Model file for the job. Use its own axes, mm. A direction names the side the tool comes from. Round coordinates to 2 decimals unless told otherwise and drop trailing zeros. Write each loop counter-clockwise with the first axis right and the second up, starting at its lowest first coordinate (ties: lowest second). Pieces come first, ordered by that corner, then holes. Notation, with made-up numbers: (16.25, 21.25) - (52.25, 21.25) arc R27 ccw to (52.25, 46.25) - close; hole circle Ø10 at (25.5, -39). An arc over 180 degrees is marked (long way). One line per item, written item: value.
from build123d import *

# Parameters (mm, degrees)
SKETCH1_W                                        = 192.5
SKETCH1_H                                        = 55
BOSS_EXTRUDE1_DEPTH                              = 20
CBORE_FOR_M4_HEX_HEAD_MACHINE_SCREW1_D           = 4.5
CBORE_FOR_M4_HEX_HEAD_MACHINE_SCREW1_DEPTH       = 55
CBORE_FOR_M4_HEX_HEAD_MACHINE_SCREW1_CBORE_D     = 9
CBORE_FOR_M4_HEX_HEAD_MACHINE_SCREW1_CBORE_DEPTH = 50
CBORE_FOR_M4_HEX_HEAD_MACHINE_SCREW2_D           = 4.5
CBORE_FOR_M4_HEX_HEAD_MACHINE_SCREW2_DEPTH       = 20
CBORE_FOR_M4_HEX_HEAD_MACHINE_SCREW2_CBORE_D     = 9
CBORE_FOR_M4_HEX_HEAD_MACHINE_SCREW2_CBORE_DEPTH = 5
CHAMFER1_SIZE                                    = 1


with BuildPart() as part:
    # Sketch1 → Boss-Extrude1 (new body)
    with BuildSketch(Plane(origin=(0, 0, 0), x_dir=(-1, 0, 0), z_dir=(0, 0, -1))):
        with Locations((-96.25, 27.5)):
            Rectangle(SKETCH1_W, SKETCH1_H)
    extrude(amount=-BOSS_EXTRUDE1_DEPTH)

    # CBORE for M4 Hex Head Machine Screw1
    with Locations(Plane(origin=(0, 0, 0), x_dir=(-1, 0, 0), z_dir=(0, -1, 0))):
        with Locations((-110, -10), (-10, -10)):
            CounterBoreHole(CBORE_FOR_M4_HEX_HEAD_MACHINE_SCREW1_D / 2, CBORE_FOR_M4_HEX_HEAD_MACHINE_SCREW1_CBORE_D / 2, CBORE_FOR_M4_HEX_HEAD_MACHINE_SCREW1_CBORE_DEPTH, depth=CBORE_FOR_M4_HEX_HEAD_MACHINE_SCREW1_DEPTH)

    # CBORE for M4 Hex Head Machine Screw2
    with Locations(Plane(origin=(0, 0, 0), x_dir=(-1, 0, 0), z_dir=(0, 0, -1))):
        with Locations((-182.5, 38), (-32.5, 38)):
            CounterBoreHole(CBORE_FOR_M4_HEX_HEAD_MACHINE_SCREW2_D / 2, CBORE_FOR_M4_HEX_HEAD_MACHINE_SCREW2_CBORE_D / 2, CBORE_FOR_M4_HEX_HEAD_MACHINE_SCREW2_CBORE_DEPTH, depth=CBORE_FOR_M4_HEX_HEAD_MACHINE_SCREW2_DEPTH)

    # Chamfer1
    chamfer1_edges = [part.edges().sort_by_distance(p)[0] for p in [
        (192.5, 27.5, 20),
        (96.25, 0, 20),
        (0, 27.5, 20),
        (96.25, 0, 0),
        (192.5, 27.5, 0),
        (96.25, 55, 0),
        (0, 27.5, 0),
        (0, 0, 10),
        (192.5, 0, 10),
        (192.5, 55, 10),
        (0, 55, 10),
        (96.25, 55, 20),
    ]]
    chamfer(chamfer1_edges, length=CHAMFER1_SIZE)


solid = part.part
1. Band-saw the part on B-B on y = 38. Write the cut outline in (x, z).
Report:
outline: (0, 1) - (1, 0) - (28, 0) - (28, 5) - (30.25, 5) - (30.25, 20) - (1, 20) - (0, 19) - close; (34.75, 5) - (37, 5) - (37, 0) - (178, 0) - (178, 5) - (180.25, 5) - (180.25, 20) - (34.75, 20) - close; (184.75, 5) - (187, 5) - (187, 0) - (191.5, 0) - (192.5, 1) - (192.5, 19) - (191.5, 20) - (184.75, 20) - close; hole circle Ø9 at (10, 10); hole circle Ø9 at (110, 10)
2. Mould opens along X. For faces 4 (the face through (98, 55, 10)), 5 (the face through (114.496, 24.65, 9.802)), 6 (the face through (192.5, 27, 10)), 7 (the face through (0, 27, 10)) say: released by +X, released by -X, zero draft, split by the parting line, or undercut.
Report:
face 4: zero draft
face 5: undercut
face 6: released by +X
face 7: released by -X
3. Band-saw the part on A-A on x = 32.5. Write the cut outline in (y, z), plus the area to 4 significant figures.
Report:
outline: (0, 1) - (1, 0) - (33.5, 0) - (33.5, 5) - (35.75, 5) - (35.75, 20) - (1, 20) - (0, 19) - close; (40.25, 5) - (42.5, 5) - (42.5, 0) - (54, 0) - (55, 1) - (55, 19) - (54, 20) - (40.25, 20) - close
area: 985.5 mm²
4. Tool access for faces 1 (the face through (33.71, 39.897, 12.605)), 2 (the face through (185, 37, 5)), 3 (the face through (8, 50, 12)): list every direction of +Z, -Z, +X, -X, +Y, -Y with a clear straight run to the whole face (end or side of a thin tool).
Report:
face 1: +Z, -Z
face 2: -Z
face 3: -Y
5. Drop flat-ended pins along their axis: pin 1 (7 mm diameter, centred on x = 183, y = 38, fed in from -Z); pin 2 (4 mm diameter, centred on x = 182.5, y = 38, fed in from +Z). Give the stop position or say it passes through.
Report:
pin 1: z = 5
pin 2: through
6. Wall check: probe 1 along X at (y, z) = (51.15, 10); probe 2 along X at (y, z) = (39.5, 4.75); probe 3 along Y at (x, z) = (182.5, 2.25). Give the ranges that are in metal, low to high. Write a range as [from, to].
Report:
probe 1: [0, 7.75], [12.25, 107.75], [112.25, 192.5]
probe 2: [0, 28.26], [36.74, 178.26], [186.74, 192.5]
probe 3: [0, 33.5], [42.5, 55]
7. Band-saw the part on C-C on z = 10. Write the cut outline in (x, y).
Report:
outline: (0, 1) - (1, 0) - (5.5, 0) - (5.5, 50) - (7.75, 50) - (7.75, 55) - (1, 55) - (0, 54) - close; (12.25, 50) - (14.5, 50) - (14.5, 0) - (105.5, 0) - (105.5, 50) - (107.75, 50) - (107.75, 55) - (12.25, 55) - close; (112.25, 50) - (114.5, 50) - (114.5, 0) - (191.5, 0) - (192.5, 1) - (192.5, 54) - (191.5, 55) - (112.25, 55) - close; hole circle Ø4.5 at (32.5, 38); hole circle Ø4.5 at (182.5, 38)
8. Band-saw the part on D-D on y = 13. Write the cut outline in (x, z), plus the area to 3 significant figures.
Report:
outline: (0, 1) - (1, 0) - (191.5, 0) - (192.5, 1) - (192.5, 19) - (191.5, 20) - (1, 20) - (0, 19) - close; hole circle Ø9 at (10, 10); hole circle Ø9 at (110, 10)
area: 3,720 mm²
